Answer from the drawing. Dimensions are ordinates in mm from the lowest x, y and z of the part. Round coordinates to 2 decimals unless told otherwise and drop trailing zeros. Loops run counter-clockwise (first coordinate to the right, second up) from the corner with the lowest first, then second, coordinate; pieces in that order, holes last.
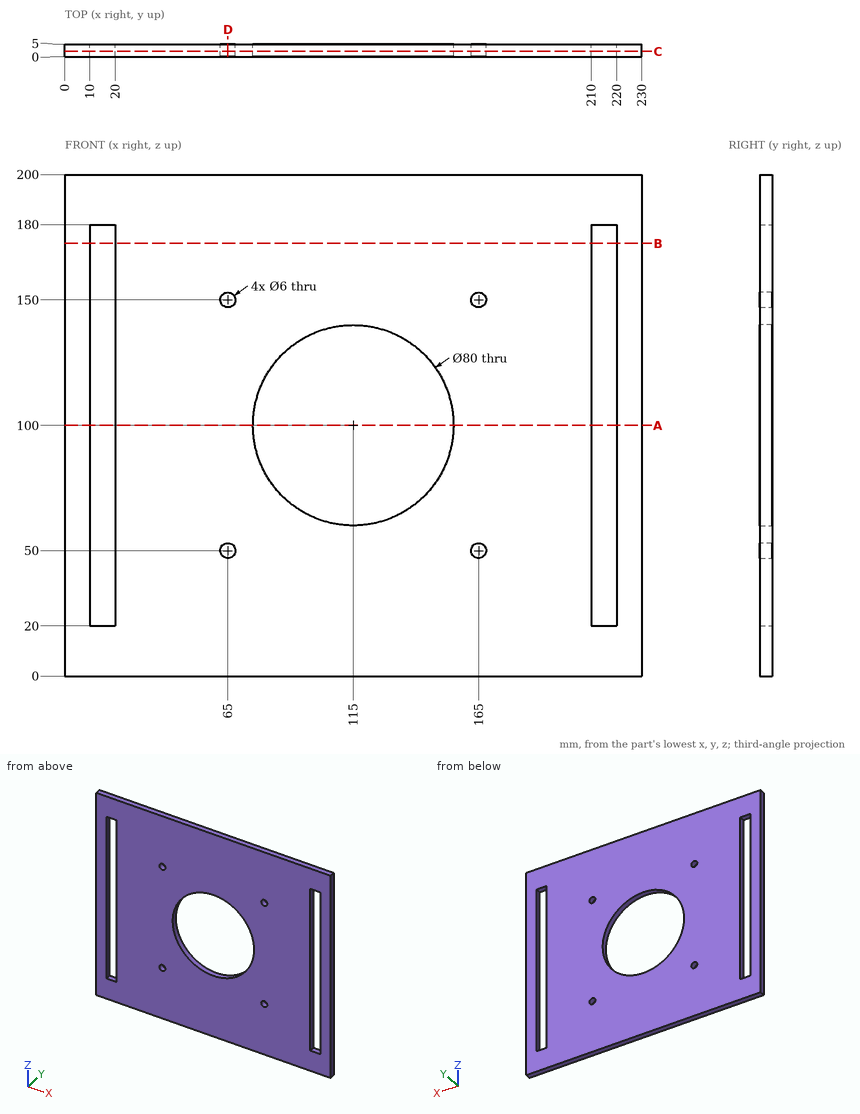
1. Find section C-C (y = 2.05). Write down the section's boundary in (x, z).
Answer key:
outline: (0, 0) - (230, 0) - (230, 200) - (0, 200) - close; hole (10, 20) - (20, 20) - (20, 180) - (10, 180) - close; hole circle Ø6 at (65, 50); hole circle Ø6 at (65, 150); hole circle Ø80 at (115, 100); hole circle Ø6 at (165, 50); hole circle Ø6 at (165, 150); hole (210, 20) - (220, 20) - (220, 180) - (210, 180) - close
2. Find section B-B (z = 172.5). Write down the section's boundary in (x, y).
Answer key:
outline: (0, 0) - (10, 0) - (10, 5) - (0, 5) - close; (20, 0) - (210, 0) - (210, 5) - (20, 5) - close; (220, 0) - (230, 0) - (230, 5) - (220, 5) - close
3. Consider probe 1 along Z at (x, y) = (165, 3); probe 2 along X at (y, z) = (3.4, 50); probe 3 along X at (y, z) = (3.15, 100). Determine where each line is inside the solid, lowest interval first.
Answer key:
probe 1: z = 0 to 47, 53 to 147, 153 to 200
probe 2: x = 0 to 10, 20 to 62, 68 to 162, 168 to 210, 220 to 230
probe 3: x = 0 to 10, 20 to 75, 155 to 210, 220 to 230
4. Find section D-D (x = 65). Write down the section's boundary in (y, z).
Answer key:
outline: (0, 0) - (5, 0) - (5, 47) - (0, 47) - close; (0, 53) - (5, 53) - (5, 147) - (0, 147) - close; (0, 153) - (5, 153) - (5, 200) - (0, 200) - close
5. Find section A-A (z = 100). Write down the section's boundary in (x, y), then the cut area to 3 significant figures.
Answer key:
outline: (0, 0) - (10, 0) - (10, 5) - (0, 5) - close; (20, 0) - (75, 0) - (75, 5) - (20, 5) - close; (155, 0) - (210, 0) - (210, 5) - (155, 5) - close; (220, 0) - (230, 0) - (230, 5) - (220, 5) - close
area: 650 mm2
